Autodesk Inventor part; units mm, degrees
ref_plane "Work Plane1" through (19.95, 0, 0) normal (1, 0, 0) x (0, 0, -1)
ref_plane "YZ Plane" through (0, 0, 0) normal (1, 0, 0) x (0, 1, 0)
ref_plane "XZ Plane" through (0, 0, 0) normal (0, 1, 0) x (-1, 0, 0)
sketch "Sketch1" plane through (0, 0, 0) normal (1, 0, 0) x (0, 1, 0)
  line L0 (0, 0) -> (2, 0)
  line L1 (6.5, 0) -> (6.5, -9)
  line L2 (6.5, -9) -> (2, -9)
  line L3 (0, -9) -> (0, 0)
  line L4 (10, 5.5) -> (2, 5.5)
  line L5 (2, 5.5) -> (2, 0)
  line L6 (2, -14.5) -> (10, -14.5)
  line L7 (10, -14.5) -> (10, 5.5)
  line L8 (10, -4.5) -> (6.5, -4.5)
  line L9 (2, 0) -> (6.5, 0)
  line L10 (2, 0) -> (2, -14.5)
  line L11 (2, -9) -> (0, -9)
  dimension "d0" = 6.5
  dimension "d1" = 9
  dimension "d3" = 10
  dimension "d4" = 20
  dimension "d5" = 2
extrude "Extrusion1" add sketch "Sketch1" along normal blind 39.9 contours L5 L4 L7 L8 L1 L9 | L2 L1 L8 L7 L6 L10
sketch "Sketch2" plane through (39.9, 0, 0) normal (1, 0, 0) x (0, 0, -1)
  line L0 (0, 6.5) -> (9, 6.5)
  line L1 (9, 6.5) -> (9, 2)
  line L2 (9, 2) -> (14.5, 2)
  line L3 (14.5, 2) -> (14.5, 10)
  line L4 (14.5, 10) -> (-5.5, 10)
  line L5 (-5.5, 10) -> (-5.5, 2)
  line L6 (-5.5, 2) -> (0, 2)
  line L7 (0, 2) -> (0, 6.5)
  line L8 (0, 5.5) -> (1.25, 4.25)
  line L9 (1.25, 4.25) -> (0, 3)
  line L10 (9, 5.5) -> (7.75, 4.25)
  line L11 (7.75, 4.25) -> (9, 3)
  line L12 (9, 6.5) -> (9, 2)
  line L13 (9, 5.5) -> (0, 5.5)
  line L14 (0, 3) -> (9, 3)
  point P0 (0, 0)
  dimension "d8" = 90
  dimension "d9" = 45
  dimension "d10" = 3.5
  dimension "d11" = 1
  dimension "d12" = 45
extrude "Extrusion2" add sketch "Sketch2" against normal up to surface (39.9 mm away) contours L8 L9 L7 | L1 L11 L10
chamfer "Chamfer1" distance 0.5 angle 45 4 edges at (19.95, 6.5, -9) (19.95, 6.5, 0) (19.95, 4.25, -1.25) (19.95, 4.25, -7.75)
sketch "Sketch3" plane through (0, 10, 5.5) normal (0, 1, 0) x (1, 0, 0)
  line L0 (0, 20) -> (0, 0)
  line L1 (0, 0) -> (39.9, 0)
  line L2 (39.9, 20) -> (39.9, 0)
  line L3 (0, 20) -> (39.9, 20)
  line L4 (0, 0) -> (39.9, 20) construction
  line L5 (27.95, 2.5) -> (11.95, 2.5)
  line L6 (11.95, 2.5) -> (11.95, 17.5)
  line L7 (11.95, 17.5) -> (27.95, 17.5)
  line L8 (27.95, 17.5) -> (27.95, 2.5)
  line L9 (27.95, 2.5) -> (11.95, 17.5) construction
  line L10 (11.95, 2.5) -> (27.95, 17.5) construction
  circle A0 centre (11.95, 17.5) radius 1.5
  circle A1 centre (27.95, 17.5) radius 1.5
  circle A2 centre (27.95, 2.5) radius 1.5
  circle A3 centre (11.95, 2.5) radius 1.5
  point P0 (0, 5.5)
  point P1 (19.95, 10)
  dimension "d18" = 16
  dimension "d19" = 15
  dimension "d20" = 3
  dimension "d21" = 3
  dimension "d22" = 3
  dimension "d23" = 3
extrude "Extrusion3" cut sketch "Sketch3" against normal blind 3 contours A3 L6 L5 | L5 L6 A3 | A2 L8 L5 | L5 L8 A2 | A0 L7 L6 | L6 L7 A0 | A1 L7 L8 | L8 L7 A1
sketch "Sketch4" plane through (0, 10, 5.5) normal (0, 1, 0) x (1, 0, 0)
  circle A0 centre (11.95, 2.5) radius 1.5
  circle A1 centre (27.95, 17.5) radius 1.5
  circle A2 centre (11.95, 17.5) radius 1.5
  circle A3 centre (27.95, 2.5) radius 1.5
  line L0 (0, 20) -> (0, 0)
  line L1 (0, 0) -> (39.9, 0)
  line L2 (39.9, 20) -> (39.9, 0)
  line L3 (0, 20) -> (39.9, 20)
  line L4 (39.9, 20) -> (39.9, 0)
  line L5 (0, 5.5) -> (39.9, 5.5)
  line L6 (39.9, 5.5) -> (39.9, 14.5)
  line L7 (39.9, 14.5) -> (0, 14.5)
  line L8 (0, 14.5) -> (0, 5.5)
  line L9 (0, 14.5) -> (39.9, 14.5)
extrude "Extrusion4" cut sketch "Sketch4" against normal blind 0.2 contours L7 L2 L5 L0
sketch "Sketch5" plane through (39.9, 0, 0) normal (1, 0, 0) x (0, 0, -1)
  line L0 (0, 9.8) -> (0, 10)
  line L1 (0, 10) -> (-5.5, 10) construction
  line L2 (-5.5, 10) -> (-5.5, 2)
  line L3 (-5.5, 2) -> (0, 2)
  line L4 (0, 2) -> (0, 3)
  line L5 (0, 3) -> (0.8964, 3.8964)
  line L6 (0.8964, 4.6036) -> (0.8964, 3.8964)
  line L7 (0.8964, 4.6036) -> (0, 5.5)
  line L8 (0, 5.5) -> (0, 6) construction
  line L9 (0.5, 6.5) -> (0, 6) construction
  line L10 (0.5, 6.5) -> (8.5, 6.5)
  line L11 (9, 6) -> (8.5, 6.5)
  line L12 (9, 6) -> (9, 5.5)
  line L13 (9, 5.5) -> (8.1036, 4.6036) construction
  line L14 (8.1036, 3.8964) -> (8.1036, 4.6036) construction
  line L15 (8.1036, 3.8964) -> (9, 3) construction
  line L16 (9, 3) -> (9, 2)
  line L17 (9, 2) -> (14.5, 2)
  line L18 (14.5, 2) -> (14.5, 10)
  line L19 (14.5, 10) -> (9, 10)
  line L20 (9, 10) -> (9, 9.8)
  line L21 (9, 9.8) -> (0, 9.8)
  line L22 (-5.25, 9.5) -> (14.25, 9.5)
  line L23 (14.25, 9.5) -> (14.25, 2)
  line L24 (14.25, 2) -> (-5.25, 2)
  line L25 (-5.25, 2) -> (-5.25, 9.5)
  circle A0 centre (4.5, 2) radius 50
  point P0 (0, 0)
  dimension "d28" = 0.25
  dimension "d29" = 0.25
  dimension "d30" = 0.5
  dimension "d31" = 100
extrude "Extrusion5" cut sketch "Sketch5" against normal blind 5
ref_plane "Work Plane1" through (19.95, 0, 0) normal (1, 0, 0) x (0, 0, -1)
mirror "Mirror1" about plane through (19.95, 0, 0) normal (1, 0, 0) of "Extrusion5"
properties part number "mgn9h_carriage"
The listing builds one solid part. Answer for the finished solid, in the listing's coordinates (mm). A direction names the side the tool comes from. Give positions to 0.01 mm unless a question says otherwise; leave off trailing zeros. Write each loop counter-clockwise with the first axis right and the second up, starting at its lowest first coordinate (ties: lowest second). Pieces come first, ordered by that corner, then holes. Notation, with made-up numbers: (30, 60.25) - (82, 60.25) arc R16 ccw to (82, 70.25) - close; hole circle Ø7 at (11, 47.25). An arc over 180 degrees is marked (long way). Use one line per item in the form item = value. Start each with the question number.
1) Consider line 1 along Z through (x, y) = (27.95, 8.35); line 2 along X through (y, z) = (8.1, -12); line 3 along Z through (x, y) = (6.5, 5.5). Determine where each line is inside the solid, lowest interval first. Write a range as from..to.
2) Flat-ended cylindrical pins translate along their axes: pin 1 Ø2.5 at (x, z) = (27.95, -12) entering from +Y; pin 2 Ø4 at (x, y) = (37, 6) entering from +Z; pin 3 Ø4 at (x, z) = (14, -4) entering from +Y. Find the tip coordinate at first contact, or state that the pin passes through.
3) Find section C-C on z = -3.25. Determine the outline of the cut face in (x, y), plus the area to 3 significant figures.
4) A tool of negligible diameter and unlimited length cuts with its end or side. For faces 4 (the face through (2, 9.5, -5)), 5 (the face through (20.2, 3.5, -0.5)), 6 (the face through (28, 7, 3)), from which of +Z, -Z, +X, -X, +Y, -Y can it reach the whole face along a straight path? Write none if from no direction.
5) Find section A-A on y = 8.5. Determine the outline of the cut face in (x, z), plus the area to 3 significant figures.
6) The mould has two halves that part along Z. Classify faces 1 (the face through (28, 7, -12)), 2 (the face through (2, 6, -14.25)), 3 (the face through (0, 7, -4)): pulls with the +Z half, pulls with the -Z half, needs draft (parallel to the pull), parting line crosses it, or undercut.
Geometry results:
q1.line_1 = -14.5..-13.5, -10.5..1.5, 4.5..5.5
q1.line_2 = 0..10.45, 13.45..26.45, 29.45..39.9
q1.line_3 = -14.5..-9, 0..5.5
q2.pin_1 = 7
q2.pin_2 = 5.25
q2.pin_3 = 9.8
q3.outline = (0, 6.5) - (39.9, 6.5) - (39.9, 9.5) - (34.9, 9.5) - (34.9, 9.8) - (5, 9.8) - (5, 9.5) - (0, 9.5) - close
q3.area = 129 mm2
q4.face_4 = +Z, -Z, -X, +Y
q4.face_5 = +X, -X, -Y
q4.face_6 = +Y
q5.outline = (0, -14.25) - (5, -14.25) - (5, -14.5) - (34.9, -14.5) - (34.9, -14.25) - (39.9, -14.25) - (39.9, 5.25) - (34.9, 5.25) - (34.9, 5.5) - (5, 5.5) - (5, 5.25) - (0, 5.25) - close; hole circle Ø3 at (11.95, -12); hole circle Ø3 at (11.95, 3); hole circle Ø3 at (27.95, -12); hole circle Ø3 at (27.95, 3)
q5.area = 765 mm2
q6.face_1 = undercut
q6.face_2 = pulls with the -Z half
q6.face_3 = needs draft
